from build123d import *

# Parameters (mm, degrees)
SKETCH1_W           = 10
SKETCH1_H           = 36.5
BOSS_EXTRUDE1_DEPTH = 12
SKETCH2_W           = 11
SKETCH2_H           = 35.5
CUT_EXTRUDE1_DEPTH  = 34.725476075
SKETCH3_R           = 1.6
CUT_EXTRUDE2_DEPTH  = 16.77
SKETCH4_R           = 1.6
CUT_EXTRUDE4_DEPTH  = 16.77
FILLET1_R           = 5
FILLET2_R           = 5
SKETCH8_W           = 5
SKETCH8_H           = 1
BOSS_EXTRUDE2_DEPTH = 6
FILLET6_R           = 2.5
SKETCH9_R           = 1.6
CUT_EXTRUDE6_DEPTH  = 1
SKETCH10_W          = 2.5
SKETCH10_H          = 5.5
CUT_EXTRUDE7_DEPTH  = 1
FILLET7_R           = 2.5


with BuildPart() as part:
    # Sketch1 → Boss-Extrude1 (new body)
    with BuildSketch(Plane.XY):
        with Locations((-13.157195709, -11.639927007)):
            Rectangle(SKETCH1_W, SKETCH1_H)
    extrude(amount=BOSS_EXTRUDE1_DEPTH)

    # Sketch2 → Cut-Extrude1 (cut, through all)
    with BuildSketch(Plane.ZY.offset(18.157195709)):
        with Locations((6.5, -11.139927007)):
            Rectangle(SKETCH2_W, SKETCH2_H)
    extrude(amount=-CUT_EXTRUDE1_DEPTH, mode=Mode.SUBTRACT)

    # Sketch3 → Cut-Extrude2 (cut)
    with BuildSketch(Plane.XY.offset(1)):
        with Locations((-13.157195709, 3.610072993)):
            Circle(SKETCH3_R)
    extrude(amount=-CUT_EXTRUDE2_DEPTH, mode=Mode.SUBTRACT)

    # Sketch4 → Cut-Extrude4 (cut)
    with BuildSketch(Plane(origin=(0, -28.889927007, 0), x_dir=(1, 0, 0), z_dir=(0, 1, 0))):
        with Locations(Location((-13.157195709, -8, 0), (0, 0, 270))):
            Circle(SKETCH4_R)
    extrude(amount=-CUT_EXTRUDE4_DEPTH, mode=Mode.SUBTRACT)

    # Fillet1
    fillet1_edges = [part.edges().sort_by_distance(p)[0] for p in [
        (-18.157195709, -29.389927007, 12),
    ]]
    fillet(fillet1_edges, radius=FILLET1_R)

    # Fillet2
    fillet2_edges = [part.edges().sort_by_distance(p)[0] for p in [
        (-8.157195709, -29.389927007, 12),
    ]]
    fillet(fillet2_edges, radius=FILLET2_R - 0.0001)  # a hair under: the kernel refuses the full size

    # Sketch8 → Boss-Extrude2 (add)
    with BuildSketch(Plane.XZ.offset(29.889927007)):
        with Locations((-13.157195709, 0.5)):
            Rectangle(SKETCH8_W, SKETCH8_H)
    extrude(amount=BOSS_EXTRUDE2_DEPTH)

    # Fillet6
    fillet6_edges = [part.edges().sort_by_distance(p)[0] for p in [
        (-15.657195709, -35.889927007, 0.5),
        (-10.657195709, -35.889927007, 0.5),
    ]]
    fillet(fillet6_edges, radius=FILLET6_R - 0.0001)  # a hair under: the kernel refuses the full size

    # Sketch9 → Cut-Extrude6 (cut)
    with BuildSketch(Plane.XY.offset(1)):
        with Locations((-13.157195709, -33.389927007)):
            Circle(SKETCH9_R)
    extrude(amount=-CUT_EXTRUDE6_DEPTH, mode=Mode.SUBTRACT)

    # Sketch10 → Cut-Extrude7 (cut)
    with BuildSketch(Plane(origin=(0, 0, 0), x_dir=(-1, 0, 0), z_dir=(0, 0, -1))):
        with Locations((9.407195709, 3.860072993)):
            Rectangle(SKETCH10_W, SKETCH10_H)
        with Locations((16.907195709, 3.860072993)):
            Rectangle(SKETCH10_W, SKETCH10_H)
    extrude(amount=-CUT_EXTRUDE7_DEPTH, mode=Mode.SUBTRACT)

    # Fillet7
    fillet7_edges = [part.edges().sort_by_distance(p)[0] for p in [
        (-10.657195709, 6.610072993, 0.5),
        (-15.657195709, 6.610072993, 0.5),
    ]]
    fillet(fillet7_edges, radius=FILLET7_R - 0.0001)  # a hair under: the kernel refuses the full size


solid = part.part
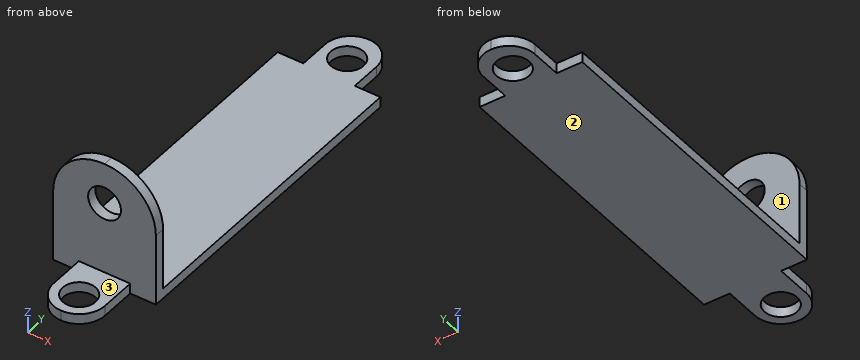
Geometry: final body of the model. Coordinates: model frame, mm. Face numbers are marked on the shaded views. A direction names the side the tool comes from. Coordinates: 2 decimals unless noted, no trailing zeros. Loops run counter-clockwise (first coordinate to the right, second up) from the corner with the lowest first, then second, coordinate; pieces in that order, holes last. Notation, with made-up numbers: M -6,-40 L 23,-40 A23 cw 23,-12 Z; hole C 25,76 d7. An arc over 180 degrees is marked long. One line per item, written item: value. Start each with the question number.
1) Cut plane C-C (y = -24.5). Return loops of the section in (x, z).
2) Reachability of the marked faces 1, 2 and 3 from +Z, -Z, +X, -X, +Y, -Y: full face, straight path, thin tool, end or side. Return the list, or none.
3) Pin query (flat end, axial travel): P1, Ø1.1, axis at y = -31, z = 0.5, coming from the +X side; P2, Ø4, axis at x = -14.5, z = 10.5, coming from the +Y side; P3, Ø5.5, axis at x = -14, y = -33, coming from the +Z side; P4, Ø2.5, axis at x = -13.16, y = -33.39, coming from the +Z side. Return the tip coordinate at first contact, or that it passes through.
4) Material intervals for L1, parallel to Y at x = -14, z = 0.5; L2, parallel to Z at x = -15.5, y = -6; L3, parallel to Y at x = -11.5, z = 3.75, sorted ascending. Write a range as from..to.
5) Cut plane D-D (z = 2.75). Return loops of the section in (x, y), then the cut area to 3 significant figures.
6) Cut plane A-A (x = -14.25). Return loops of the section in (y, z).
7) Cut plane B-B (z = 8). Return loops of the section in (x, y), then the cut area to 3 significant figures.
Evaluation:
1. outline: M -18.16,0 L -8.16,0 L -8.16,1 L -18.16,1 Z
2. face 1: +Z, +X, -X, +Y
2. face 2: -Z, +X, -X, +Y, -Y
2. face 3: +Z, +X, -X, -Y
3. P1: x = -10.66
3. P2: y = -28.89
3. P3: z = 1
3. P4: through
4. L1: -35.74..-34.75, -32.03..2.25, 4.97..6.46
4. L2: 0..1
4. L3: -29.89..-28.89
5. outline: M -18.16,-29.89 L -8.16,-29.89 L -8.16,-28.89 L -18.16,-28.89 Z
5. area: 10.0 mm^2
6. outline: M -35.64,0 L -34.56,0 L -34.56,1 L -35.64,1 Z; M -32.22,0 L 2.44,0 L 2.44,1 L -28.89,1 L -28.89,6.83 L -29.89,6.83 L -29.89,1 L -32.22,1 Z; M -29.89,9.17 L -28.89,9.17 L -28.89,11.88 L -29.89,11.88 Z; M 4.78,0 L 6.36,0 L 6.36,1 L 4.78,1 Z
7. outline: M -18.06,-29.89 L -14.76,-29.89 L -14.76,-28.89 L -18.06,-28.89 Z; M -11.56,-29.89 L -8.26,-29.89 L -8.26,-28.89 L -11.56,-28.89 Z
7. area: 6.60 mm^2
